Geometry: final body of the model. Coordinates: model frame, mm. A direction names the side the tool comes from. Coordinates: 2 decimals unless noted, no trailing zeros. Loops run counter-clockwise (first coordinate to the right, second up) from the corner with the lowest first, then second, coordinate; pieces in that order, holes last. Notation, with made-up numbers: M -3,20.25 L 2,20.25 A15 ccw 2,36.25 Z; hole C 34,27.5 d6. An arc over 180 degrees is marked long. Write item = value, one per line. Start each with the question number.
```python
from build123d import *

# Parameters (mm, degrees)
SKETCH1_W           = 88.9
SKETCH1_H           = 71.12
BOSS_EXTRUDE1_DEPTH = 1.778
SKETCH2_R           = 1.524
CUT_EXTRUDE1_DEPTH  = 2.54
BOSS_EXTRUDE2_DEPTH = 19.05
CUT_EXTRUDE2_START  = -1.778
CUT_EXTRUDE2_DEPTH  = 1.778
BOSS_EXTRUDE3_DEPTH = 2.54
BOSS_EXTRUDE4_DEPTH = 3.81
BOSS_EXTRUDE5_DEPTH = 1.778
SKETCH10_W          = 19.05
SKETCH10_H          = 9.906
CUT_EXTRUDE5_DEPTH  = 1.778
SKETCH12_W          = 8.128
SKETCH12_H          = 2.54
CUT_EXTRUDE6_DEPTH  = 8.509
SKETCH14_R          = 1.27
CUT_EXTRUDE7_DEPTH  = 3.81


with BuildPart() as part:
    # Sketch1 → Boss-Extrude1 (new body)
    with BuildSketch(Plane.XY):
        Rectangle(SKETCH1_W, SKETCH1_H)
    extrude(amount=BOSS_EXTRUDE1_DEPTH)

    # Sketch2 → Cut-Extrude1 (cut)
    with BuildSketch(Plane(origin=(0, 0, 0), x_dir=(-1, 0, 0), z_dir=(0, 0, -1))):
        with Locations((-42.344998858, 22.278284854)):
            Circle(SKETCH2_R)
        with Locations((42.344998858, 22.278284854)):
            Circle(SKETCH2_R)
        with Locations((41.275, -32.385)):
            Circle(SKETCH2_R)
        with Locations((-41.275, -32.385)):
            Circle(SKETCH2_R)
    extrude(amount=-CUT_EXTRUDE1_DEPTH, mode=Mode.SUBTRACT)

    # Sketch3 → Boss-Extrude2 (add)
    with BuildSketch(Plane.XY.offset(1.778)):
        with BuildLine():
            Line((-20.982004201, 0.529316706), (-20.982004201, -27.156683294))
            ThreePointArc((-20.982004201, -27.156683294), (-20.461240058, -28.413919151), (-19.204004201, -28.934683294))
            Line((-19.204004201, -28.934683294), (37.945995799, -28.934683294))
            ThreePointArc((37.945995799, -28.934683294), (39.203231656, -28.413919151), (39.723995799, -27.156683294))
            Line((39.723995799, -27.156683294), (39.723995799, 0.529316706))
            ThreePointArc((39.723995799, 0.529316706), (39.203231656, 1.786552563), (37.945995799, 2.307316706))
            Line((37.945995799, 2.307316706), (-19.204004201, 2.307316706))
            ThreePointArc((-19.204004201, 2.307316706), (-20.461240058, 1.786552563), (-20.982004201, 0.529316706))
        make_face()
        with BuildLine():
            Line((-19.204004201, -1.248683294), (-19.204004201, -25.378683294))
            ThreePointArc((-19.204004201, -25.378683294), (-18.683240058, -26.635919151), (-17.426004201, -27.156683294))
            Line((-17.426004201, -27.156683294), (36.167995799, -27.156683294))
            ThreePointArc((36.167995799, -27.156683294), (37.425231656, -26.635919151), (37.945995799, -25.378683294))
            Line((37.945995799, -25.378683294), (37.945995799, -1.248683294))
            ThreePointArc((37.945995799, -1.248683294), (37.425231656, 0.008552563), (36.167995799, 0.529316706))
            Line((36.167995799, 0.529316706), (-17.426004201, 0.529316706))
            ThreePointArc((-17.426004201, 0.529316706), (-18.683240058, 0.008552563), (-19.204004201, -1.248683294))
        make_face(mode=Mode.SUBTRACT)
    extrude(amount=BOSS_EXTRUDE2_DEPTH)

    # Sketch4 → Cut-Extrude2 (cut)
    with BuildSketch(Plane.XY.offset(1.778).offset(CUT_EXTRUDE2_START)):
        with BuildLine():
            Line((-17.426004201, 0.529316706), (36.167995799, 0.529316706))
            ThreePointArc((36.167995799, 0.529316706), (37.425231656, 0.008552563), (37.945995799, -1.248683294))
            Line((37.945995799, -1.248683294), (37.945995799, -25.378683294))
            ThreePointArc((37.945995799, -25.378683294), (37.425231656, -26.635919151), (36.167995799, -27.156683294))
            Line((36.167995799, -27.156683294), (-17.426004201, -27.156683294))
            ThreePointArc((-17.426004201, -27.156683294), (-18.683240058, -26.635919151), (-19.204004201, -25.378683294))
            Line((-19.204004201, -25.378683294), (-19.204004201, -1.248683294))
            ThreePointArc((-19.204004201, -1.248683294), (-18.683240058, 0.008552563), (-17.426004201, 0.529316706))
        make_face()
    extrude(amount=CUT_EXTRUDE2_DEPTH, mode=Mode.SUBTRACT)

    # Sketch5 → Boss-Extrude3 (add)
    with BuildSketch(Plane.XY.offset(1.778)):
        with BuildLine():
            Line((-12.845316988, 2.307316706), (-4.717316988, 2.307316706))
            ThreePointArc((-4.717316988, 2.307316706), (-8.781316988, 6.371316706), (-12.845316988, 2.307316706))
        make_face()
        with BuildLine():
            Line((31.587308585, 2.307316706), (23.459308585, 2.307316706))
            ThreePointArc((23.459308585, 2.307316706), (27.523308585, 6.371316706), (31.587308585, 2.307316706))
        make_face()
        with BuildLine():
            Line((5.306995799, -28.934683294), (13.434995799, -28.934683294))
            ThreePointArc((13.434995799, -28.934683294), (9.370995799, -32.998683294), (5.306995799, -28.934683294))
        make_face()
    extrude(amount=BOSS_EXTRUDE3_DEPTH)

    # Sketch6 → Boss-Extrude4 (add)
    with BuildSketch(Plane.XY.offset(4.318)):
        with BuildLine():
            Line((5.306995799, -28.934683294), (13.434995799, -28.934683294))
            ThreePointArc((13.434995799, -28.934683294), (9.370995799, -32.998683294), (5.306995799, -28.934683294))
        make_face()
    extrude(amount=BOSS_EXTRUDE4_DEPTH)

    # Sketch7 → Boss-Extrude5 (add)
    with BuildSketch(Plane.XY.offset(20.828)):
        with BuildLine():
            Line((-19.204004201, 2.307316706), (37.945995799, 2.307316706))
            ThreePointArc((37.945995799, 2.307316706), (39.203231656, 1.786552563), (39.723995799, 0.529316706))
            Line((39.723995799, 0.529316706), (39.723995799, -27.156683294))
            ThreePointArc((39.723995799, -27.156683294), (39.203231656, -28.413919151), (37.945995799, -28.934683294))
            Line((37.945995799, -28.934683294), (-19.204004201, -28.934683294))
            ThreePointArc((-19.204004201, -28.934683294), (-20.461240058, -28.413919151), (-20.982004201, -27.156683294))
            Line((-20.982004201, -27.156683294), (-20.982004201, 0.529316706))
            ThreePointArc((-20.982004201, 0.529316706), (-20.461240058, 1.786552563), (-19.204004201, 2.307316706))
        make_face()
    extrude(amount=BOSS_EXTRUDE5_DEPTH)

    # Sketch10 → Cut-Extrude5 (cut)
    with BuildSketch(Plane.ZY.offset(20.982004201)):
        with Locations((11.303, -13.313683294)):
            Rectangle(SKETCH10_W, SKETCH10_H)
    extrude(amount=-CUT_EXTRUDE5_DEPTH, mode=Mode.SUBTRACT)

    # Sketch12 → Cut-Extrude6 (cut, symmetric)
    with BuildSketch(Plane(origin=(0, 2.307316706, 0), x_dir=(1, 0, 0), z_dir=(0, 1, 0))):
        with Locations((-8.781316988, -3.048)):
            Rectangle(SKETCH12_W, SKETCH12_H)
        with Locations((27.523308585, -3.048)):
            Rectangle(SKETCH12_W, SKETCH12_H)
    extrude(amount=CUT_EXTRUDE6_DEPTH, both=True, mode=Mode.SUBTRACT)

    # Sketch14 → Cut-Extrude7 (cut)
    with BuildSketch(Plane(origin=(0, 0, 0), x_dir=(-1, 0, 0), z_dir=(0, 0, -1))):
        with Locations((-9.370995799, -29.824748275)):
            Circle(SKETCH14_R)
    extrude(amount=-CUT_EXTRUDE7_DEPTH, mode=Mode.SUBTRACT)


solid = part.part
```
Item 1: Reachability of faces 5 (the flat face through (-20, -18.267, 11)), 6 (the cylindrical face through (-20.447, -28.428, 12.046)), 7 (the flat face through (9, 0.529, 10)), 8 (the flat face through (-12.845, 1, 3)), 9 (the flat face through (10, -28.935, 12)) from +Z, -Z, +X, -X, +Y, -Y: full face, straight path, thin tool, end or side. Return the list, or none.
Item 2: Section query C-C (z = 12.25). Return the cut outline in (x, y).
Item 3: Line query: line 1 (X direction, y = -20, z = 18.5); line 2 (Y direction, x = -15.5, z = 9.5); line 3 (Y direction, x = 6.5, z = 21). Output: solid intervals per line, ascending. Write a range as from..to.
Item 4: Section query D-D (y = 27.5). Return the cut outline in (x, z).
Item 5: Section query A-A (x = 33). Return the cut outline in (y, z).
Item 6: Section query B-B (y = -16). Return the cut outline in (x, z), plus the area to 3 significant figures.
Item 7: First-contact query: pin 1 (10 mm diameter, centred on x = 16.5, y = 10.5, fed in from +Z); pin 2 (6 mm diameter, centred on x = 21.5, z = 14.5, fed in from +Y); pin 3 (0.5 mm diameter, centred on x = -20, z = 15, fed in from +Y); pin 4 (2.5 mm diameter, centred on x = 42.34, y = 22.28, fed in from -Z). Flat tips, straight axial feed; report the tip coordinate or a pass-through.
Item 8: Pull-direction query (X, two-part tool) for faces 1 (the flat face through (9, -30, 8.128)), 2 (the cylindrical face through (9.46, -32.998, 4.909)), 3 (the flat face through (-4.717, 1, 3)), 4 (the cylindrical face through (-20.475, 1.773, 12.046)); classes: released by +X, released by -X, zero draft, split by the parting line, or undercut.
Verdict:
q1.face_5 = -X
q1.face_6 = +Z, -X, -Y
q1.face_7 = -Z
q1.face_8 = +Y
q1.face_9 = +Z, -Y
q2.outline = M -20.98,-27.16 A1.78 ccw -19.2,-28.93 L 37.95,-28.93 A1.78 ccw 39.72,-27.16 L 39.72,0.53 A1.78 ccw 37.95,2.31 L -19.2,2.31 A1.78 ccw -20.98,0.53 L -20.98,-8.36 L -19.2,-8.36 L -19.2,-1.25 A1.78 cw -17.43,0.53 L 36.17,0.53 A1.78 cw 37.95,-1.25 L 37.95,-25.38 A1.78 cw 36.17,-27.16 L -17.43,-27.16 A1.78 cw -19.2,-25.38 L -19.2,-18.27 L -20.98,-18.27 Z
q3.line_1 = -20.98..-19.2, 37.95..39.72
q3.line_2 = -28.93..-27.16, 0.53..2.31
q3.line_3 = -28.93..2.31
q4.outline = M -44.45,0 L 44.45,0 L 44.45,1.78 L -44.45,1.78 Z
q5.outline = M -35.56,0 L -27.16,0 L -27.16,20.83 L 0.53,20.83 L 0.53,0 L 35.56,0 L 35.56,1.78 L 2.31,1.78 L 2.31,22.61 L -28.93,22.61 L -28.93,1.78 L -35.56,1.78 Z
q6.outline = M -44.45,0 L -19.2,0 L -19.2,1.78 L -44.45,1.78 Z; M -20.98,20.83 L 37.95,20.83 L 37.95,0 L 44.45,0 L 44.45,1.78 L 39.72,1.78 L 39.72,22.61 L -20.98,22.61 Z
q6.area = 198 mm2
q7.pin_1 = 1.78
q7.pin_2 = 2.31
q7.pin_3 = 2.22
q7.pin_4 = through
q8.face_1 = zero draft
q8.face_2 = split by the parting line
q8.face_3 = undercut
q8.face_4 = released by -X
